```python
from build123d import *

# Parameters (mm, degrees)
F3_R     = 2.8468654953
F4_DEPTH = 133.5461065173
F5_R     = 5.6267762556
F6_DEPTH = 35.052


with BuildPart() as f1:
    # F0 (on Front) → F1 (revolve)
    with BuildSketch(Plane.XZ):
        with BuildLine():
            Line((-3.6975557381, 9.2503800988), (-63.8671591878, 9.2503800988))
            Line((-63.8671591878, 9.2503800988), (-63.8671591878, 5.3283213638))
            Line((-63.8671591878, 5.3283213638), (-4.4152569437, 5.3283213638))
            ThreePointArc((-4.4152569437, 5.3283213638), (-1.0384074547, 6.3006464453), (1.3043017336, 8.9198528508))
            ThreePointArc((1.3043017336, 8.9198528508), (18.3668266982, 19.6340703482), (35.4293516628, 8.9198528508))
            ThreePointArc((35.4293516628, 8.9198528508), (37.772060851, 6.3006464453), (41.14891034, 5.3283213638))
            Line((41.14891034, 5.3283213638), (69.6789473295, 5.3283213638))
            Line((69.6789473295, 5.3283213638), (69.6789473295, 9.2503800988))
            Line((69.6789473295, 9.2503800988), (40.4312091344, 9.2503800988))
            ThreePointArc((40.4312091344, 9.2503800988), (37.4422386518, 9.9978310848), (35.1569245265, 12.0642209007))
            ThreePointArc((35.1569245265, 12.0642209007), (18.3668266982, 21.02176981), (1.5767288699, 12.0642209007))
            ThreePointArc((1.5767288699, 12.0642209007), (-0.7085852554, 9.9978310848), (-3.6975557381, 9.2503800988))
        make_face()
    revolve(axis=Axis((-34.1412080657, 0, 5.3283213638), (1, 0, 0)))

    # F3 (on face) → F4 (cut, through all)
    with BuildSketch(Plane.YZ.offset(69.6789473295)):
        with Locations((0, 5.2630640566)):
            Circle(F3_R)
    extrude(amount=-F4_DEPTH, mode=Mode.SUBTRACT)

    # F5 (on Top) → F6 (cut)
    with BuildSketch(Plane.XY):
        with Locations((18.277015537, 0)):
            Circle(F5_R)
    extrude(amount=F6_DEPTH, mode=Mode.SUBTRACT)


solid = f1.part
```
Design review of the part built by this model. Coordinates are the model's own, in mm. A direction names the side the tool comes from. Round coordinates to 2 decimals unless told otherwise and drop trailing zeros. Answer in a Markdown table with one row per item.
Q1. Draft analysis for pull direction Y (two halves, no side actions). For faces 1 (the face through (69.679, -3, 6)), 2 (the face through (52.982, -0.371, 8.086)), 3 (the face through (-34.204, 1.502, 8.951)), state which applies: +Y half, -Y half, draft (parallel to the pull), parting line (faces both ways), or undercut.
The answers:
| item | result |
|---|---|
| face 1 | draft |
| face 2 | undercut |
| face 3 | parting line |
Q2. Clearance check with flat-ended pins moving along their axes: pin 1 Ø3 at (y, z) = (5, 5.5) entering from +X; pin 2 Ø3 at (x, y) = (-19.5, 1) entering from -Z; pin 3 Ø3 at (x, y) = (5, -8) entering from -Z; pin 4 Ø4.5 at (y, z) = (0, 5.26) entering from +X. State where each tip first meets the part, or that it passes through.
The answers:
| item | result |
|---|---|
| pin 1 | x = 69.68 |
| pin 2 | z = 1.41 |
| pin 3 | z = -3.87 |
| pin 4 | through |
Q3. To check wall thickness, follow L1, parallel to Z at x = 48, y = 0; L2, parallel to Y at x = -11.5, z = 5; L3, parallel to Y at x = 31.5, z = 3. State the ranges of each line that lie inside material, in increasing order. Write a range as [from, to].
The answers:
| item | result |
|---|---|
| L1 | [1.41, 2.42], [8.11, 9.25] |
| L2 | [-3.91, -2.83], [2.83, 3.91] |
| L3 | [-10.59, -8.71], [8.71, 10.59] |
Q4. For faces 4 (the face through (54.85, 1.502, 8.951)), 5 (the face through (-31.018, -0.371, 8.086)), 6 (the face through (17.057, -5.493, 19.352)), list the 3-axis set-ups (+Z, -Z, +X, -X, +Y, -Y) from which the entire face can be reached by the end or side of a thin tool; tool diameter is ignored.
The answers:
| item | result |
|---|---|
| face 4 | +X |
| face 5 | +X, -X |
| face 6 | +Z |
Q5. Take a section at A-A, the plane y = 0. Count the separate pieces of the cut face and the enclosed holes in it, then the cut area to 3 significant figures.
The answers:
| item | result |
|---|---|
| separate pieces | 3 |
| enclosed holes | 0 |
| area | 326 mm² |
